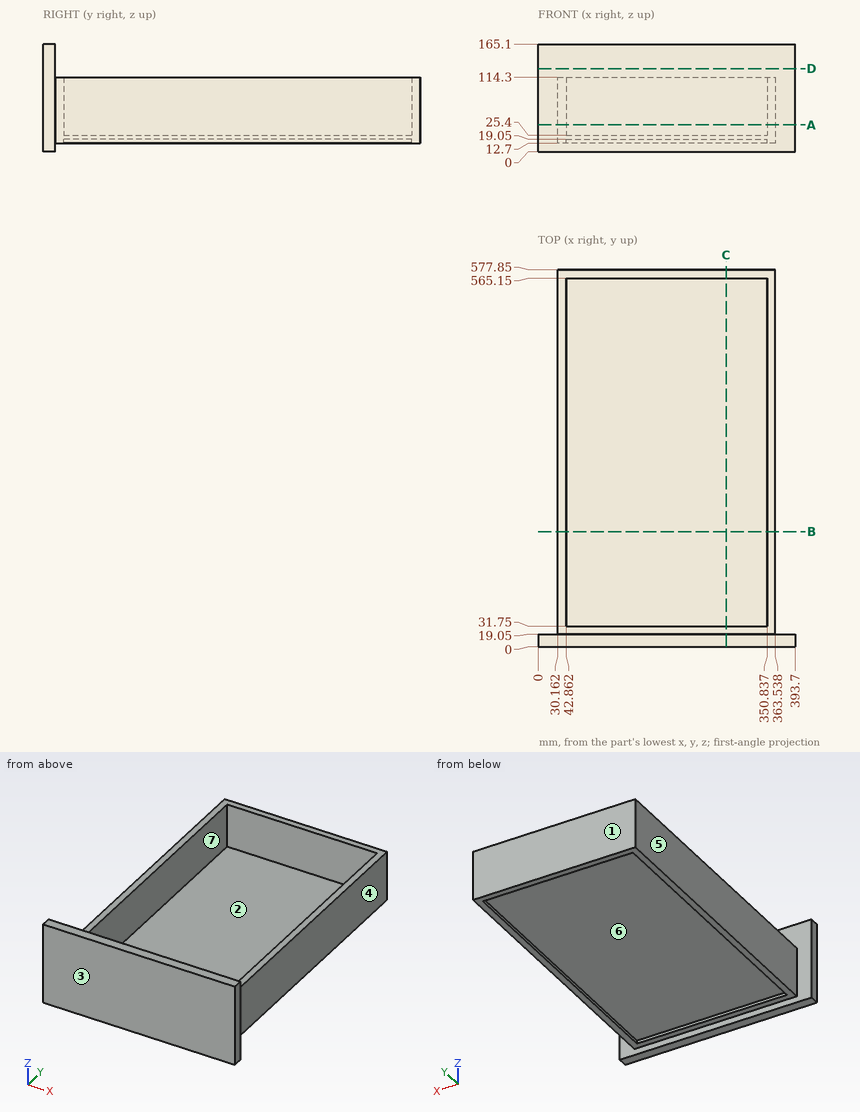
The figure shows three views and two pictorial views of one solid part (mm, origin at its lowest corner). Answer the questions. A direction names the side the tool comes from. Give positions to 0.01 mm unless a question says otherwise; leave off trailing zeros. Loops run counter-clockwise (first coordinate to the right, second up) from the corner with the lowest first, then second, coordinate; pieces in that order, holes last. Notation, with made-up numbers: M -21.5,-7.5 L 29.5,-7.5 A28 ccw 29.5,20.5 Z; hole C 31.25,69 d3. An arc over 180 degrees is marked long. Write each question's results on one line, items separated by ' | '.
1. Section C-C on x = 288 is taken. Give the vertices of the cut face in (y, z), plus the area to 3 significant figures.
Values:
outline: M 0,0 L 19.05,0 L 19.05,12.7 L 31.75,12.7 L 31.75,19.05 L 565.15,19.05 L 565.15,12.7 L 577.85,12.7 L 577.85,114.3 L 565.15,114.3 L 565.15,25.4 L 31.75,25.4 L 31.75,114.3 L 19.05,114.3 L 19.05,165.1 L 0,165.1 Z | area: 9,110 mm^2
2. Straight lines are drawn through the part: line 1 (Y direction, x = 341, z = 109); line 2 (X direction, y = 182.5, z = 15); line 3 (Z direction, x = 93, y = 548.5). For each, find the intervals that lie inside material, in ascending order. Write a range as [from, to].
Values:
line 1: y = [0, 31.75], [565.15, 577.85] | line 2: x = [30.16, 42.86], [350.84, 363.54] | line 3: z = [19.05, 25.4]
3. Given pin 1 (1.9 mm diameter, centred on y = 223, z = 15.5, fed in from -X); pin 2 (1.5 mm diameter, centred on x = 202.5, y = 482, fed in from +Z); pin 3 (1.5 mm diameter, centred on x = 290.5, z = 125, fed in from +Y), each flat-ended and moving along its own axis, determine where each tip first touches the part or whether it passes through.
Values:
pin 1: stops at x = 30.16 | pin 2: stops at z = 25.4 | pin 3: stops at y = 19.05
4. Section B-B on y = 176.5 is taken. Give the vertices of the cut face in (x, z), plus the area to 3 significant figures.
Values:
outline: M 30.16,12.7 L 42.86,12.7 L 42.86,19.05 L 350.84,19.05 L 350.84,12.7 L 363.54,12.7 L 363.54,114.3 L 350.84,114.3 L 350.84,25.4 L 42.86,25.4 L 42.86,114.3 L 30.16,114.3 Z | area: 4,540 mm^2
5. The mould has two halves that part along Y. Classify the marked faces 1, 2, 3 and 4: pulls with the +Y half, pulls with the -Y half, needs draft (parallel to the pull), parting line crosses it, or undercut.
Values:
face 1: pulls with the +Y half | face 2: undercut | face 3: pulls with the -Y half | face 4: needs draft
6. Section A-A on z = 41 is taken. Give the vertices of the cut face in (x, y), plus the area to 3 significant figures.
Values:
outline: M 0,0 L 393.7,0 L 393.7,19.05 L 363.54,19.05 L 363.54,577.85 L 30.16,577.85 L 30.16,19.05 L 0,19.05 Z; hole M 42.86,31.75 L 350.84,31.75 L 350.84,565.15 L 42.86,565.15 Z | area: 29,500 mm^2
7. A tool of negligible diameter and unlimited length cuts with its end or side. For the marked faces 5, 6 and 7, from which of +Z, -Z, +X, -X, +Y, -Y can it reach the whole face along a straight path? Write none if from no direction.
Values:
face 5: +Z, -Z, -X, +Y | face 6: -Z | face 7: +Z
8. Section D-D on z = 127.5 is taken. Give the vertices of the cut face in (x, y).
Values:
outline: M 0,0 L 393.7,0 L 393.7,19.05 L 0,19.05 Z
